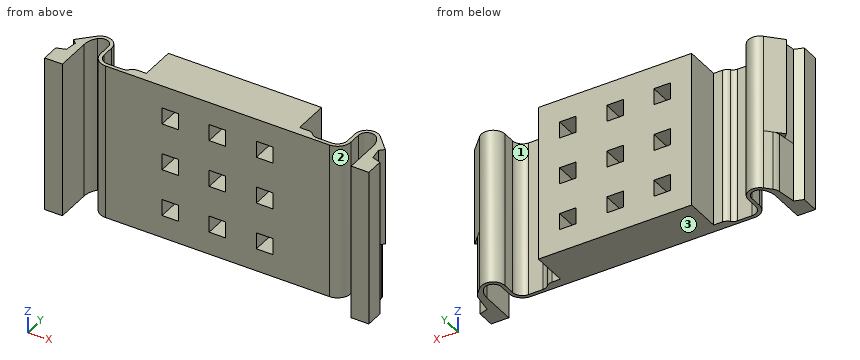
```python
from build123d import *

# Parameters (mm, degrees)
RESSALTO_EXTRUS_O1_DEPTH = 16.5
ESBO_O4_W                = 1.5
ESBO_O4_H                = 16.5
RESSALTO_EXTRUS_O2_DEPTH = 2
RESSALTO_EXTRUS_O3_START = -10
RESSALTO_EXTRUS_O3_DEPTH = 10
ESBO_O5_W                = 26
ESBO_O5_H                = 26.5
RESSALTO_EXTRUS_O4_DEPTH = 6
ESBO_O6_W                = 2.8
ESBO_O6_H                = 2.8
CORTE_EXTRUS_O1_DEPTH    = 33.058488003
RESSALTO_EXTRUS_O5_DEPTH = 26.5


with BuildPart() as part:
    # Esboço3 → Ressalto-extrusão1 (new body)
    with BuildSketch(Plane.XY):
        with BuildLine():
            Line((18.985114218, -0.6), (-18.983112061, -0.6))
            ThreePointArc((-18.983112061, -0.6), (-20.575873515, 0.059743396), (-21.235616911, 1.65250485))
            Line((-21.235616911, 1.65250485), (-21.235616911, 3.729745078))
            ThreePointArc((-21.235616911, 3.729745078), (-22.112654073, 5.030006142), (-23.646779042, 4.703917814))
            ThreePointArc((-23.646779042, 4.703917814), (-24.278856787, 3.652335225), (-24.498998922, 2.44532004))
            Line((-24.498998922, 2.44532004), (-24.498998922, -1.5))
            Line((-24.498998922, -1.5), (-25.998998922, -1.5))
            Line((-25.998998922, -1.5), (-25.998998922, 0))
            Line((-25.998998922, 0), (-25.72065272, 1.980536137))
            Line((-25.72065272, 1.980536137), (-26.43999252, 2.675194508))
            Line((-26.43999252, 2.675194508), (-24.078382922, 5.120712836))
            ThreePointArc((-24.078382922, 5.120712836), (-21.887890117, 5.586316455), (-20.635616911, 3.729745078))
            Line((-20.635616911, 3.729745078), (-20.635616911, 1.65250485))
            ThreePointArc((-20.635616911, 1.65250485), (-20.151609446, 0.484007465), (-18.983112061, 0))
            Line((-18.983112061, 0), (-16.483112061, 0))
            ThreePointArc((-16.483112061, 0), (-15.962423979, 0.111330278), (-15.532789063, 0.425852691))
            ThreePointArc((-15.532789063, 0.425852691), (-15.049887248, 0.77937015), (-14.464643335, 0.904503352))
            Line((-14.464643335, 0.904503352), (-7.266260975, 0.904503352))
            Line((-7.266260975, 0.904503352), (7.268263132, 0.904503352))
            Line((7.268263132, 0.904503352), (14.466645491, 0.904503352))
            ThreePointArc((14.466645491, 0.904503352), (15.051889405, 0.77937015), (15.53479122, 0.425852691))
            ThreePointArc((15.53479122, 0.425852691), (15.964426136, 0.111330278), (16.485114218, 0))
            Line((16.485114218, 0), (18.985114218, 0))
            ThreePointArc((18.985114218, 0), (20.153611603, 0.484007465), (20.637619068, 1.65250485))
            Line((20.637619068, 1.65250485), (20.637619068, 3.729745078))
            ThreePointArc((20.637619068, 3.729745078), (21.889892273, 5.586316455), (24.080385079, 5.120712836))
            Line((24.080385079, 5.120712836), (26.441994677, 2.675194508))
            Line((26.441994677, 2.675194508), (25.722654876, 1.980536137))
            Line((25.722654876, 1.980536137), (26.001001078, 0))
            Line((26.001001078, 0), (26.001001078, -1.5))
            Line((26.001001078, -1.5), (24.501001078, -1.5))
            Line((24.501001078, -1.5), (24.501001078, 2.44532004))
            ThreePointArc((24.501001078, 2.44532004), (24.280858943, 3.652335225), (23.648781199, 4.703917814))
            ThreePointArc((23.648781199, 4.703917814), (22.11465623, 5.030006142), (21.237619068, 3.729745078))
            Line((21.237619068, 3.729745078), (21.237619068, 1.65250485))
            ThreePointArc((21.237619068, 1.65250485), (20.577875672, 0.059743396), (18.985114218, -0.6))
        make_face()
    extrude(amount=RESSALTO_EXTRUS_O1_DEPTH)

    # Esboço4 → Ressalto-extrusão2 (add)
    with BuildSketch(Plane.XZ.offset(1.5)):
        with Locations((25.251001078, 8.25)):
            Rectangle(ESBO_O4_W, ESBO_O4_H)
        with Locations((-25.248998922, 8.25)):
            Rectangle(ESBO_O4_W, ESBO_O4_H)
    extrude(amount=RESSALTO_EXTRUS_O2_DEPTH)

    # Esboço2 → Ressalto-extrusão3 (add)
    with BuildSketch(Plane.XY.offset(RESSALTO_EXTRUS_O3_START)):
        with BuildLine():
            Line((14.466645491, 0.904503352), (-14.464643335, 0.904503352))
            ThreePointArc((-14.464643335, 0.904503352), (-15.049887248, 0.77937015), (-15.532789063, 0.425852691))
            ThreePointArc((-15.532789063, 0.425852691), (-15.962423979, 0.111330278), (-16.483112061, 0))
            Line((-16.483112061, 0), (-18.983112061, 0))
            ThreePointArc((-18.983112061, 0), (-20.151609446, 0.484007465), (-20.635616911, 1.65250485))
            Line((-20.635616911, 1.65250485), (-20.635616911, 3.729745078))
            ThreePointArc((-20.635616911, 3.729745078), (-21.887890117, 5.586316455), (-24.078382922, 5.120712836))
            Line((-24.078382922, 5.120712836), (-25.082936671, 4.080466977))
            ThreePointArc((-25.082936671, 4.080466977), (-25.400658676, 3.626789441), (-25.562720122, 3.09716064))
            Line((-25.562720122, 3.09716064), (-25.998998922, 0))
            Line((-25.998998922, 0), (-25.998998922, -3.5))
            Line((-25.998998922, -3.5), (-24.498998922, -3.5))
            Line((-24.498998922, -3.5), (-24.498998922, 2.44532004))
            ThreePointArc((-24.498998922, 2.44532004), (-24.278856787, 3.652335225), (-23.646779042, 4.703917814))
            ThreePointArc((-23.646779042, 4.703917814), (-22.112654073, 5.030006142), (-21.235616911, 3.729745078))
            Line((-21.235616911, 3.729745078), (-21.235616911, 1.65250485))
            ThreePointArc((-21.235616911, 1.65250485), (-20.575873515, 0.059743396), (-18.983112061, -0.6))
            Line((-18.983112061, -0.6), (18.985114218, -0.6))
            ThreePointArc((18.985114218, -0.6), (20.577875672, 0.059743396), (21.237619068, 1.65250485))
            Line((21.237619068, 1.65250485), (21.237619068, 3.729745078))
            ThreePointArc((21.237619068, 3.729745078), (22.11465623, 5.030006142), (23.648781199, 4.703917814))
            ThreePointArc((23.648781199, 4.703917814), (24.280858943, 3.652335225), (24.501001078, 2.44532004))
            Line((24.501001078, 2.44532004), (24.501001078, -3.5))
            Line((24.501001078, -3.5), (26.001001078, -3.5))
            Line((26.001001078, -3.5), (26.001001078, 0))
            Line((26.001001078, 0), (25.564722279, 3.09716064))
            ThreePointArc((25.564722279, 3.09716064), (25.402660833, 3.626789441), (25.084938828, 4.080466977))
            Line((25.084938828, 4.080466977), (24.080385079, 5.120712836))
            ThreePointArc((24.080385079, 5.120712836), (21.889892273, 5.586316455), (20.637619068, 3.729745078))
            Line((20.637619068, 3.729745078), (20.637619068, 1.65250485))
            ThreePointArc((20.637619068, 1.65250485), (20.153611603, 0.484007465), (18.985114218, 0))
            Line((18.985114218, 0), (16.485114218, 0))
            ThreePointArc((16.485114218, 0), (15.964426136, 0.111330278), (15.53479122, 0.425852691))
            ThreePointArc((15.53479122, 0.425852691), (15.051889405, 0.77937015), (14.466645491, 0.904503352))
        make_face()
    extrude(amount=RESSALTO_EXTRUS_O3_DEPTH)

    # Esboço5 → Ressalto-extrusão4 (add)
    with BuildSketch(Plane(origin=(0, 0.904503352, 0), x_dir=(1, 0, 0), z_dir=(0, 1, 0))):
        with Locations((0.001001078, -3.25)):
            Rectangle(ESBO_O5_W, ESBO_O5_H)
    extrude(amount=RESSALTO_EXTRUS_O4_DEPTH)

    # Esboço6 → Corte-extrusão1 (cut, through all)
    with BuildSketch(Plane.XZ.offset(0.6)):
        with Locations((0.001001078, 11.25)):
            Rectangle(ESBO_O6_W, ESBO_O6_H)
        with Locations((-7.998998922, 11.25)):
            Rectangle(ESBO_O6_W, ESBO_O6_H)
        with Locations((8.001001078, 11.25)):
            Rectangle(ESBO_O6_W, ESBO_O6_H)
        with Locations((0.001001078, 3.25)):
            Rectangle(ESBO_O6_W, ESBO_O6_H)
        with Locations((8.001001078, 3.25)):
            Rectangle(ESBO_O6_W, ESBO_O6_H)
        with Locations((0.001001078, -4.75)):
            Rectangle(ESBO_O6_W, ESBO_O6_H)
        with Locations((8.001001078, -4.75)):
            Rectangle(ESBO_O6_W, ESBO_O6_H)
        with Locations((-7.998998922, 3.25)):
            Rectangle(ESBO_O6_W, ESBO_O6_H)
        with Locations((-7.998998922, -4.75)):
            Rectangle(ESBO_O6_W, ESBO_O6_H)
    extrude(amount=-CORTE_EXTRUS_O1_DEPTH, mode=Mode.SUBTRACT)

    # Esboço8 → Ressalto-extrusão5 (add, through all)
    with BuildSketch(Plane.XY.offset(16.5)):
        Polygon((-25.998998922, -3.5), (-27.498998922, -3.5), (-27.498998922, -0.5), (-25.998998922, 0), align=None)
        Polygon((26.001001078, 0), (26.001001078, -3.5), (27.501001078, -3.5), (27.501001078, -0.5), align=None)
    extrude(amount=-RESSALTO_EXTRUS_O5_DEPTH)


solid = part.part
```
CAD build for the part. Positions are in the model's coordinates, mm. Face numbers are marked on the shaded views. A direction names the side the tool comes from. Coordinates: 2 decimals unless noted, no trailing zeros. Order: outer loops, then holes, each group sorted by start corner. A loop starts at its lowest first (then second) coordinate and runs counter-clockwise, first axis right, second up. Notation, with made-up numbers: (-16, -11) - (-3, -11) arc R15 cw to (-3, 8) - close; hole circle Ø7 at (-21.5, 76.25). An arc over 180 degrees is marked (long way). Use a Markdown table: item, result. Add a question column.
(1) Saw through at B-B (x = 8). Give the cut face in (y, z).
(2) Flat gauge pins, fed straight in: pin 1 (12 mm diameter, centred on x = 8, z = 4.5, fed in from +Y); pin 2 (3 mm diameter, centred on y = 2.5, z = -4, fed in from +X); pin 3 (4 mm diameter, centred on x = 11, z = -1.5, fed in from -Y); pin 4 (2 mm diameter, centred on y = 3, z = -5, fed in from +X). Where does each tip first touch, or does it go through?
(3) Saw through at A-A (y = -2.5). Give the cut face in (x, z).
(4) Saw through at C-C (z = 11.5). Count the separate pieces of the cut face and the enclosed holes in it, then the cut area to 3 significant figures.
(5) Saw through at D-D (x = -12.5). Give the cut face in (y, z), then the cut area to 3 significant figures.
(6) Drill centre lines: line 1 along X through (y, z) = (4.25, 0.25); line 2 along X through (y, z) = (-2, 3.5); line 3 along X through (y, z) = (1.5, -0.25). Where is each one in solid material? Low to high. Write a range as [from, to].
(7) Which spindle directions (+Z, -Z, +X, -X, +Y, -Y) get a long thin tool onto all of the face, cutting with end or side? Do the marked faces 1, 2 and 3. Say none if no direction does.
Solved:
| question | item | result |
|---|---|---|
| 1 | outline | (-0.6, -10) - (6.9, -10) - (6.9, -6.15) - (-0.6, -6.15) - close; (-0.6, -3.35) - (6.9, -3.35) - (6.9, 1.85) - (-0.6, 1.85) - close; (-0.6, 4.65) - (6.9, 4.65) - (6.9, 9.85) - (-0.6, 9.85) - close; (-0.6, 12.65) - (6.9, 12.65) - (6.9, 16.5) - (-0.6, 16.5) - close |
| 2 | pin 1 | stops at y = 6.9 |
| 2 | pin 2 | stops at x = 25.86 |
| 2 | pin 3 | stops at y = -0.6 |
| 2 | pin 4 | stops at x = 25.72 |
| 3 | outline | (-27.5, -10) - (-24.5, -10) - (-24.5, 16.5) - (-27.5, 16.5) - close; (24.5, -10) - (27.5, -10) - (27.5, 16.5) - (24.5, 16.5) - close |
| 4 | separate pieces | 4 |
| 4 | enclosed holes | 0 |
| 4 | area | 188 mm² |
| 5 | outline | (-0.6, -10) - (6.9, -10) - (6.9, 16.5) - (-0.6, 16.5) - close |
| 5 | area | 199 mm² |
| 6 | line 1 | x = [-24.92, -23.98], [-21.34, -20.7], [-13, 13], [20.71, 21.34], [23.99, 24.92] |
| 6 | line 2 | x = [-27.5, -24.5], [24.5, 27.5] |
| 6 | line 3 | x = [-25.79, -24.5], [-21.23, -20.63], [-13, 13], [20.63, 21.23], [24.5, 25.79] |
| 7 | face 1 | +Z, -Z, +Y |
| 7 | face 2 | +Z, -Z, -Y |
| 7 | face 3 | -Z, +X, -X, +Y, -Y |
